from build123d import *

# Parameters (mm, degrees)
BOSS_EXTRUDE1_DEPTH     = 35
CUT_EXTRUDE2_DEPTH      = 21
CUT_EXTRUDE2_DEPTH_BACK = 4
BOSS_EXTRUDE2_DEPTH     = 35
SKETCH5_W               = 30
SKETCH5_H               = 25
CUT_EXTRUDE3_DEPTH      = 20
SKETCH6_R               = 2
CUT_EXTRUDE4_DEPTH      = 27


with BuildPart() as part:
    # Sketch1 → Boss-Extrude1 (new body)
    with BuildSketch(Plane.XY):
        Polygon((0, 23), (0, 0), (56, 0), (56, 3), (26, 3), (26, 23), (23, 23), (23, 3), (3, 3), (3, 23), align=None)
    extrude(amount=BOSS_EXTRUDE1_DEPTH)

    # Sketch3 → Cut-Extrude2 (cut, two sides)
    with BuildSketch(Plane(origin=(0, 3, 0), x_dir=(1, 0, 0), z_dir=(0, 1, 0))) as cut_extrude2_sk:
        with BuildLine():
            Line((31, -9.5), (51, -9.5))
            ThreePointArc((51, -9.5), (52.5, -11), (51, -12.5))
            Line((51, -12.5), (31, -12.5))
            ThreePointArc((31, -12.5), (29.5, -11), (31, -9.5))
        make_face()
        with BuildLine():
            Line((31, -25.5), (51, -25.5))
            ThreePointArc((51, -25.5), (52.5, -24), (51, -22.5))
            Line((51, -22.5), (31, -22.5))
            ThreePointArc((31, -22.5), (29.5, -24), (31, -25.5))
        make_face()
    extrude(amount=CUT_EXTRUDE2_DEPTH, mode=Mode.SUBTRACT)
    extrude(cut_extrude2_sk.sketch, amount=-CUT_EXTRUDE2_DEPTH_BACK, mode=Mode.SUBTRACT)

    # Sketch4 → Boss-Extrude2 (add, through all)
    with BuildSketch(Plane.XY.offset(35)):
        Polygon((26, 23), (26, 3), (56, 3), align=None)
    extrude(amount=-BOSS_EXTRUDE2_DEPTH)

    # Sketch5 → Cut-Extrude3 (cut)
    with BuildSketch(Plane(origin=(0, 23, 0), x_dir=(1, 0, 0), z_dir=(0, 1, 0))):
        with Locations((41, -17.5)):
            Rectangle(SKETCH5_W, SKETCH5_H)
    extrude(amount=-CUT_EXTRUDE3_DEPTH, mode=Mode.SUBTRACT)

    # Sketch6 → Cut-Extrude4 (cut, through all)
    with BuildSketch(Plane(origin=(26, 0, 0), x_dir=(0, 0, -1), z_dir=(1, 0, 0))):
        with Locations((-23.75, 13)):
            Circle(SKETCH6_R)
        with Locations((-11.25, 13)):
            Circle(SKETCH6_R)
    extrude(amount=-CUT_EXTRUDE4_DEPTH, mode=Mode.SUBTRACT)


solid = part.part
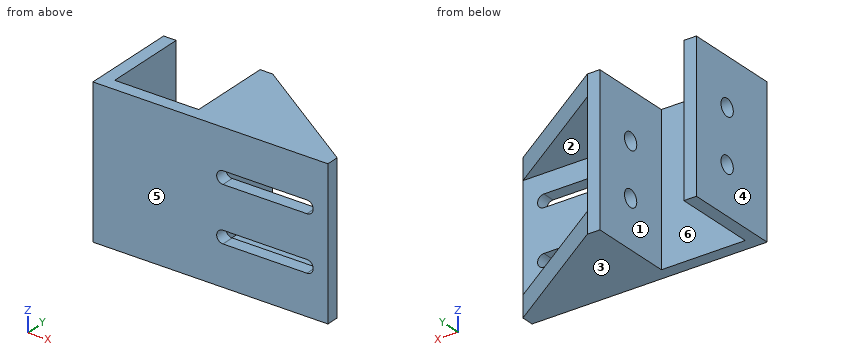
Part model, mm, in its own coordinate system. Face numbers are marked on the shaded views. A direction names the side the tool comes from. Coordinates: 2 decimals unless noted, no trailing zeros. Write each loop counter-clockwise with the first axis right and the second up, starting at its lowest first coordinate (ties: lowest second). Pieces come first, ordered by that corner, then holes. Notation, with made-up numbers: (0, 20.5) - (30, 20.5) arc R14 cw to (30, 32.5) - close; hole circle Ø8 at (-11.75, 22.25). An arc over 180 degrees is marked (long way). Put each result on its own line as item: value.
1. 3-axis set-ups, long thin cutter, end or side, ignore diameter. For the marked faces 1, 2 and 3: which of +Z, -Z, +X, -X, +Y, -Y reach the whole face in a straight line?
Final values:
face 1: +Z, -Z, +Y
face 2: +X, +Y
face 3: -Z, +X, -X, +Y, -Y
2. Band-saw the part on C-C (y = 19.5). Write the cut outline in (x, z).
Final values:
outline: (0, 0) - (3, 0) - (3, 35) - (0, 35) - close; (23, 0) - (31.25, 0) - (31.25, 5) - (26, 5) - (26, 30) - (31.25, 30) - (31.25, 35) - (23, 35) - close
3. Probe line 1 along Y through (x, z) = (1.35, 23.75); line 2 along X through (y, z) = (15.5, 21); line 3 along Z through (x, y) = (30.5, 4.25). List the from-to ranges inside material, lowest first. Write a range as [from, to].
Final values:
line 1: y = [0, 11], [15, 23]
line 2: x = [0, 3], [23, 26]
line 3: z = [0, 5], [30, 35]
4. Flat gauge pins, fed straight in: pin 1 Ø6.5 at (y, z) = (13, 23.75) entering from +X; pin 2 Ø12.5 at (x, z) = (36, 20) entering from +Y. Where does each tip first touch, or does it go through?
Final values:
pin 1: stops at x = 26
pin 2: stops at y = 3
5. Band-saw the part on A-A (x = 35). Write the cut outline in (y, z).
Final values:
outline: (0, 0) - (17, 0) - (17, 5) - (3, 5) - (3, 9.5) - (0, 9.5) - close; (0, 12.5) - (3, 12.5) - (3, 22.5) - (0, 22.5) - close; (0, 25.5) - (3, 25.5) - (3, 30) - (17, 30) - (17, 35) - (0, 35) - close
6. Band-saw the part on D-D (z = 8.5). Write the cut outline in (x, y).
Final values:
outline: (0, 0) - (56, 0) - (56, 3) - (26, 3) - (26, 23) - (23, 23) - (23, 3) - (3, 3) - (3, 23) - (0, 23) - close
7. Two-plate mould, pull along X, no slides. Class the marked faces 4, 5 and 6: +X half, -X half, draft (parallel to the pull), parting line (faces both ways), or undercut.
Final values:
face 4: -X half
face 5: draft
face 6: undercut
8. Band-saw the part on B-B (y = 13). Write the cut outline in (x, z).
Final values:
outline: (0, 0) - (3, 0) - (3, 9.25) - (0, 9.25) - close; (0, 13.25) - (3, 13.25) - (3, 21.75) - (0, 21.75) - close; (0, 25.75) - (3, 25.75) - (3, 35) - (0, 35) - close; (23, 0) - (41, 0) - (41, 5) - (26, 5) - (26, 9.25) - (23, 9.25) - close; (23, 13.25) - (26, 13.25) - (26, 21.75) - (23, 21.75) - close; (23, 25.75) - (26, 25.75) - (26, 30) - (41, 30) - (41, 35) - (23, 35) - close
